Could you check a few things on this drawing? It's one solid part, dimensions in mm from its lowest x, y, z. A direction names the side the tool comes from. Give positions to 0.01 mm unless a question says otherwise; leave off trailing zeros. Order: outer loops, then holes, each group sorted by start corner. A loop starts at its lowest first (then second) coordinate and runs counter-clockwise, first axis right, second up. Notation, with made-up numbers: M 24.25,-6 L 40.25,-6 A18 cw 40.25,7 Z; hole C -33,-4.75 d6. An arc over 180 degrees is marked long. Use CSV: the item, a comma, the result in double quotes. Start each with the question number.
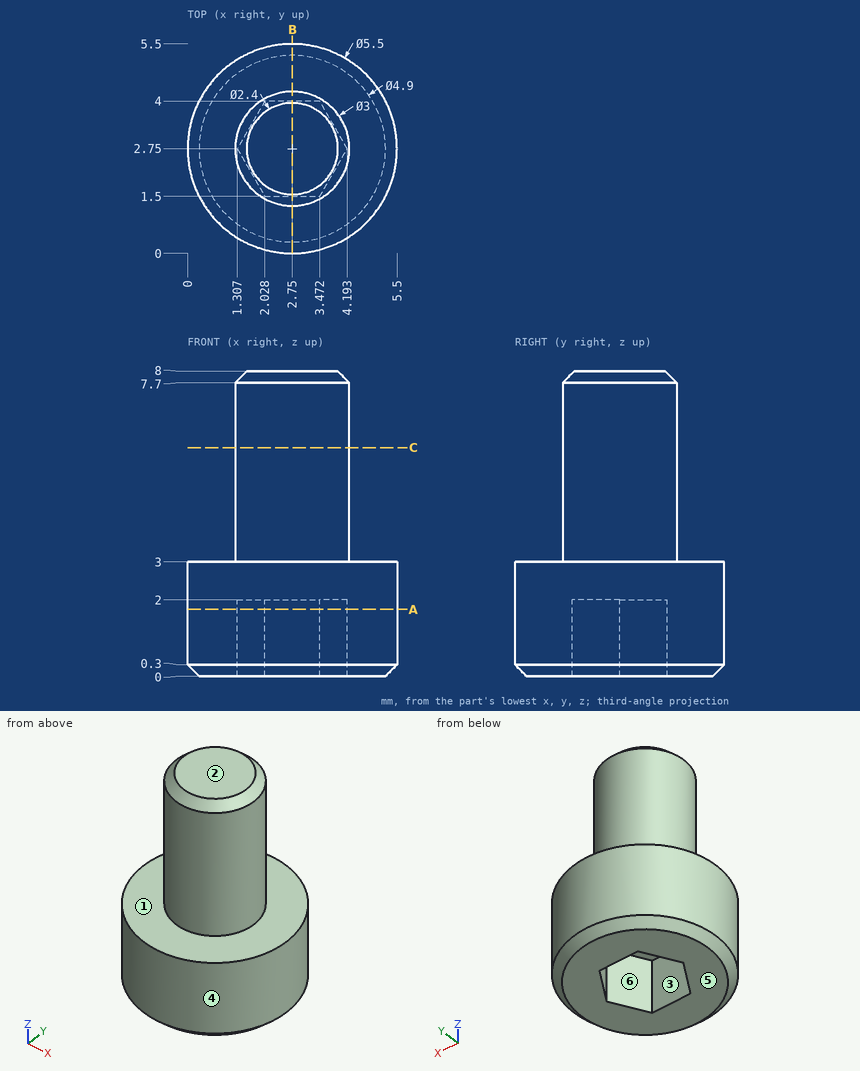
Q1. For P1, Ø2, axis at y = 4.5, z = 6, coming from the +X side; P2, Ø2, axis at y = 3.5, z = 6, coming from the +X side, each with a flat end and sliding along its axis, tell me the tip position at first contact or that it passes through.
Q2. Imagine slicing it at A-A, the plane z = 1.75. Please give me the cut outline in (x, y).
Q3. Imagine slicing it at C-C, the plane z = 6. Please give me the cut outline in (x, y).
Q4. For the marked faces 1 and 2, which set-ups out of +Z, -Z, +X, -X, +Y, -Y let a thin tool reach every point of the face, with its end or its side?
Q5. We'd pull the mould along Y, two halves only. Please class the marked faces 3, 4, 5 and 6: pulls with the +Y half, pulls with the -Y half, needs draft (parallel to the pull), parting line crosses it, or undercut.
Q6. I need wall thicknesses on line 1 (Z direction, x = 2.8, y = 4.85); line 2 (Y direction, x = 3.05, z = 4); line 3 (Z direction, x = 0.25, y = 1.85) (1 decimal). Which ranges of each line are inside material? Lowest first, please. Write a range as [from, to].
Q7. Imagine slicing it at B-B, the plane x = 2.75. Please give me the cut outline in (y, z).
Reply:
1,P1,"stops at x = 4.05"
1,P2,"stops at x = 4.25"
2,outline,"C 2.75,2.75 d5.5; hole M 1.31,2.75 L 2.03,1.5 L 3.47,1.5 L 4.19,2.75 L 3.47,4 L 2.03,4 Z"
3,outline,"C 2.75,2.75 d3"
4,face 1,"+Z"
4,face 2,"+Z, +X, -X, +Y, -Y"
5,face 3,"undercut"
5,face 4,"parting line crosses it"
5,face 5,"needs draft"
5,face 6,"undercut"
6,line 1,"z = [0, 3]"
6,line 2,"y = [1.28, 4.22]"
6,line 3,"z = [0.2, 3]"
7,outline,"M 0,0.3 L 0.3,0 L 1.5,0 L 1.5,2 L 4,2 L 4,0 L 5.2,0 L 5.5,0.3 L 5.5,3 L 4.25,3 L 4.25,7.7 L 3.95,8 L 1.55,8 L 1.25,7.7 L 1.25,3 L 0,3 Z"
